The listing builds one solid part. Answer for the finished solid, in the listing's coordinates (mm). A direction names the side the tool comes from. Round coordinates to 2 decimals unless told otherwise and drop trailing zeros. Order: outer loops, then holes, each group sorted by start corner. A loop starts at its lowest first (then second) coordinate and runs counter-clockwise, first axis right, second up. Notation, with made-up numbers: (21.5, -13) -> (26.5, -13) arc R7 ccw to (26.5, -1) -> close; hole circle Ø8 at (76, 2). An arc over 180 degrees is marked (long way). Return JSON: item names as keys, results as strings. Group by question number.
(1) This flat-tipped pin is pushed along its axis until it touches: pin 1 (10 mm diameter, centred on x = -22.5, y = -21, fed in from -Z). Where does it stop, or does it pass through?
(2) The part is cut by section C-C (x = -3.25). Determine the outline of the cut face in (y, z).
(3) The part is cut by section B-B (z = 95.5). Determine the outline of the cut face in (x, y).
(4) Determine the mould class of faces 1 (the face through (-0.906, -16.712, 6.245)), 2 (the face through (-16.72, -24.43, 93.154)), 3 (the face through (-12.53, -24.43, 16.83)) for opening direction X: +X half, -X half, draft (parallel to the pull), parting line (faces both ways), or undercut.
(5) The part is cut by section A-A (y = -6.75). Determine the outline of the cut face in (x, z).
(6) Consider line 1 (X direction, y = -10, z = 50); line 2 (Y direction, x = -18.75, z = 6); line 3 (Z direction, x = -17, y = -0.75). Determine where each line is inside the solid, lowest interval first. Write a range as [from, to].
(7) The part is cut by section D-D (z = 74). Determine the outline of the cut face in (x, y).
(8) Which of the six approach directions +Z, -Z, +X, -X, +Y, -Y give full straight-line access (tool end or side, diameter ignored) to faces 4 (the face through (-24.72, -16.2, 27.46)), 5 (the face through (-11, -1.207, 52))?
from build123d import *

# Parameters (mm, degrees)
F0_W      = 25.4
F0_H      = 25.4
F1_DEPTH  = 101.6
F2_W      = 22.225
F2_H      = 22.225
F3_DEPTH  = 101.6
F4_R      = 3.174802
F5_DEPTH  = 25.4
F6_R      = 3.175
F7_DEPTH  = 25.4
F8_R      = 3.175
F9_DEPTH  = 25.4
F10_R     = 3.175
F11_DEPTH = 25.4
F12_R     = 3.175
F13_DEPTH = 25.4
F14_R     = 3.175
F15_DEPTH = 25.4
F16_R     = 3.175
F17_DEPTH = 25.4
F18_R     = 3.175
F19_DEPTH = 25.4
F20_R     = 3.175
F21_DEPTH = 25.4
F22_R     = 3.175
F23_DEPTH = 25.4


with BuildPart() as f1:
    # F0 (on Top) → F1 (new body)
    with BuildSketch(Plane.XY):
        with Locations((-12.7, -12.7)):
            Rectangle(F0_W, F0_H)
    extrude(amount=F1_DEPTH)

    # F2 (on face) → F3 (cut)
    with BuildSketch(Plane.XY.offset(101.6)):
        with Locations((-12.899866, -12.319956)):
            Rectangle(F2_W, F2_H)
    extrude(amount=-F3_DEPTH, mode=Mode.SUBTRACT)

    # F4 (on face) → F5 (cut)
    with BuildSketch(Plane(origin=(-25.4, 0, 0), x_dir=(0, -1, 0), z_dir=(-1, 0, 0))):
        with Locations((13.779499, 7.461248)):
            Circle(F4_R)
    extrude(amount=-F5_DEPTH, mode=Mode.SUBTRACT)

    # F6 (on face) → F7 (cut)
    with BuildSketch(Plane(origin=(-25.4, 0, 0), x_dir=(0, -1, 0), z_dir=(-1, 0, 0))):
        with Locations((13.171837, 26.501355)):
            Circle(F6_R)
    extrude(amount=-F7_DEPTH, mode=Mode.SUBTRACT)

    # F8 (on face) → F9 (cut)
    with BuildSketch(Plane(origin=(-25.4, 0, 0), x_dir=(0, -1, 0), z_dir=(-1, 0, 0))):
        with Locations((12.4406, 45.537316)):
            Circle(F8_R)
    extrude(amount=-F9_DEPTH, mode=Mode.SUBTRACT)

    # F10 (on face) → F11 (cut)
    with BuildSketch(Plane(origin=(-25.4, 0, 0), x_dir=(0, -1, 0), z_dir=(-1, 0, 0))):
        with Locations((11.275698, 64.551666)):
            Circle(F10_R)
    extrude(amount=-F11_DEPTH, mode=Mode.SUBTRACT)

    # F12 (on face) → F13 (cut)
    with BuildSketch(Plane(origin=(-25.4, 0, 0), x_dir=(0, -1, 0), z_dir=(-1, 0, 0))):
        with Locations((13.80254, 83.433339)):
            Circle(F12_R)
    extrude(amount=-F13_DEPTH, mode=Mode.SUBTRACT)

    # F14 (on face) → F15 (cut)
    with BuildSketch(Plane.XZ.offset(25.4)):
        with Locations((-15.557501, 15.875)):
            Circle(F14_R)
    extrude(amount=-F15_DEPTH, mode=Mode.SUBTRACT)

    # F16 (on face) → F17 (cut)
    with BuildSketch(Plane.XZ.offset(25.4)):
        with Locations((-12.04097, 34.59762)):
            Circle(F16_R)
    extrude(amount=-F17_DEPTH, mode=Mode.SUBTRACT)

    # F18 (on face) → F19 (cut)
    with BuildSketch(Plane.XZ.offset(25.4)):
        with Locations((-14.264603, 53.517397)):
            Circle(F18_R)
    extrude(amount=-F19_DEPTH, mode=Mode.SUBTRACT)

    # F20 (on face) → F21 (cut)
    with BuildSketch(Plane.XZ.offset(25.4)):
        with Locations((-10.92981, 72.27324)):
            Circle(F20_R)
    extrude(amount=-F21_DEPTH, mode=Mode.SUBTRACT)

    # F22 (on face) → F23 (cut)
    with BuildSketch(Plane.XZ.offset(25.4)):
        with Locations((-14.380366, 91.008132)):
            Circle(F22_R)
    extrude(amount=-F23_DEPTH, mode=Mode.SUBTRACT)


solid = f1.part
Answer below:
{
 "1": {"pin 1": "stops at z = 0"},
 "2": {"outline": "(-25.4, 0) -> (-23.43, 0) -> (-23.43, 101.6) -> (-25.4, 101.6) -> close; (-1.21, 0) -> (0, 0) -> (0, 101.6) -> (-1.21, 101.6) -> close"},
 "3": {"outline": "(-25.4, -25.4) -> (0, -25.4) -> (0, 0) -> (-25.4, 0) -> close; hole (-24.01, -23.43) -> (-1.79, -23.43) -> (-1.79, -1.21) -> (-24.01, -1.21) -> close"},
 "4": {"face 1": "draft", "face 2": "undercut", "face 3": "undercut"},
 "5": {"outline": "(-25.4, 0) -> (-24.01, 0) -> (-24.01, 101.6) -> (-25.4, 101.6) -> close; (-1.79, 0) -> (0, 0) -> (0, 101.6) -> (-1.79, 101.6) -> close"},
 "6": {"line 1": "x = [-25.4, -24.01], [-1.79, 0]", "line 2": "y = [-25.4, -23.43], [-1.21, 0]", "line 3": "z = [0, 13.05], [18.7, 51.91], [55.13, 89.21], [92.8, 101.6]"},
 "7": {"outline": "(-25.4, -25.4) -> (-13.59, -25.4) -> (-13.59, -23.43) -> (-24.01, -23.43) -> (-24.01, -1.21) -> (-13.59, -1.21) -> (-13.59, 0) -> (-25.4, 0) -> close; (-8.27, -25.4) -> (0, -25.4) -> (0, 0) -> (-8.27, 0) -> (-8.27, -1.21) -> (-1.79, -1.21) -> (-1.79, -23.43) -> (-8.27, -23.43) -> close"},
 "8": {"face 4": "+X, -X", "face 5": "+Z, -Z"}
}
